Geometry check sheet. Reference: drawing and pictorial views, mm from the part's lowest x, y, z. Coordinates: 2 decimals unless noted, no trailing zeros. Write each loop counter-clockwise with the first axis right and the second up, starting at its lowest first coordinate (ties: lowest second). Pieces come first, ordered by that corner, then holes.
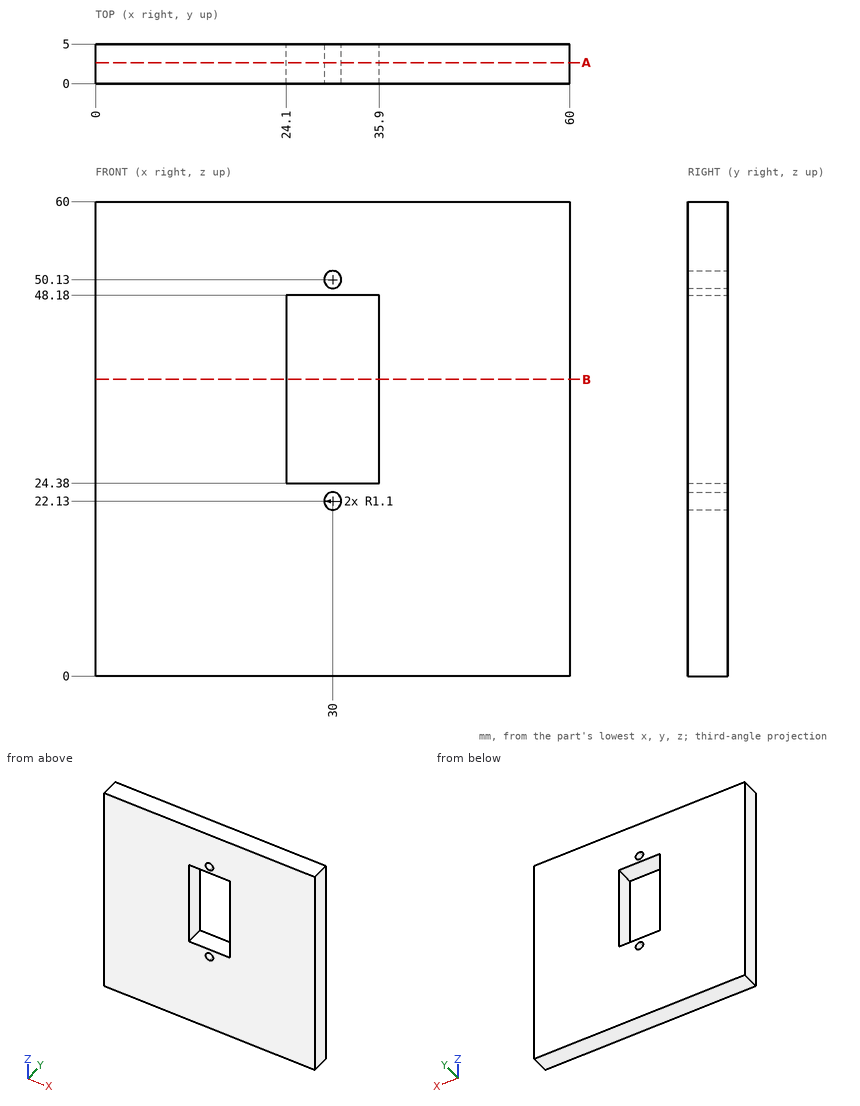
1. Sectioned sample at B-B, the plane z = 37.5. Record the boundary of the cut face in (x, y), and give its area (3 significant figures).
2. Sectioned sample at A-A, the plane y = 2.65. Record the boundary of the cut face in (x, z).
3. Material ranges on L1, parallel to X at y = 3.9, z = 48; L2, parallel to Z at x = 26, y = 2.6; L3, parallel to X at y = 0.8, z = 50.5, recorded low to high.
Outcome:
1. outline: (0, 0) - (24.1, 0) - (24.1, 5) - (0, 5) - close; (35.9, 0) - (60, 0) - (60, 5) - (35.9, 5) - close
1. area: 241 mm2
2. outline: (0, 0) - (60, 0) - (60, 60) - (0, 60) - close; hole (24.1, 24.38) - (35.9, 24.38) - (35.9, 48.18) - (24.1, 48.18) - close; hole circle Ø2.2 at (30, 22.13); hole circle Ø2.2 at (30, 50.13)
3. L1: x = 0 to 24.1, 35.9 to 60
3. L2: z = 0 to 24.38, 48.18 to 60
3. L3: x = 0 to 28.96, 31.04 to 60
